```python
from build123d import *

# Parameters (mm, degrees)
SKETCH1_W           = 190
SKETCH1_H           = 29
BOSS_EXTRUDE1_DEPTH = 3
SKETCH2_W           = 190
SKETCH2_H           = 3
BOSS_EXTRUDE2_DEPTH = 3
SKETCH3_W           = 190
SKETCH3_H           = 3
BOSS_EXTRUDE3_DEPTH = 19
SKETCH4_R           = 4.4
BOSS_EXTRUDE4_DEPTH = 190
FILLET1_R           = 1
SKETCH5_W           = 24.6
SKETCH5_H           = 9.5
SKETCH5_W_2         = 22.8
SKETCH5_W_3         = 49.2
CUT_EXTRUDE1_DEPTH  = 99.13898308
CUT_EXTRUDE3_REACH  = 100.139
SKETCH8_R           = 0.79375
CUT_EXTRUDE4_REACH  = 100.139
SKETCH9_W           = 10.2
SKETCH9_H           = 16
DRAFT1_ANGLE        = -5
FILLET2_R           = 5
FILLET3_R           = 2
SKETCH10_R          = 0.79375
BOSS_EXTRUDE5_DEPTH = 3
BOSS_EXTRUDE8_START = -190
SKETCH10_3_R        = 1.75
BOSS_EXTRUDE8_DEPTH = 3
SKETCH12_W          = 26.262284607
SKETCH12_H          = 3
SKETCH12_W_2        = 34.475430786
SKETCH12_W_3        = 52.524569214
CUT_EXTRUDE5_DEPTH  = 105.761807039
SKETCH13_R          = 4.242640687
BOSS_EXTRUDE9_DEPTH = 0.4
FILLET4_R           = 4


with BuildPart() as part:
    # Sketch1 → Boss-Extrude1 (new body)
    with BuildSketch(Plane.XY):
        Rectangle(SKETCH1_W, SKETCH1_H)
    extrude(amount=BOSS_EXTRUDE1_DEPTH)

    # Sketch2 → Boss-Extrude2 (add)
    with BuildSketch(Plane.XY.offset(3)):
        with Locations((0, 13)):
            Rectangle(SKETCH2_W, SKETCH2_H)
    extrude(amount=BOSS_EXTRUDE2_DEPTH)

    # Sketch3 → Boss-Extrude3 (add)
    with BuildSketch(Plane.XY.offset(3)):
        with Locations((0, -13)):
            Rectangle(SKETCH3_W, SKETCH3_H)
    extrude(amount=BOSS_EXTRUDE3_DEPTH)

    # Sketch4 → Boss-Extrude4 (add)
    with BuildSketch(Plane.ZY.offset(95)):
        with Locations((18.5, -9.4)):
            Circle(SKETCH4_R)
    extrude(amount=-BOSS_EXTRUDE4_DEPTH)

    # Fillet1
    fillet1_edges = [part.edges().sort_by_distance(p)[0] for p in [
        (0, -11.5, 14.633477014),
    ]]
    fillet(fillet1_edges, radius=FILLET1_R)

    # Sketch5 → Cut-Extrude1 (cut, through all)
    with BuildSketch(Plane.XY.offset(3)):
        with Locations((-82.7, -9.75)):
            Rectangle(SKETCH5_W, SKETCH5_H)
        with Locations((-47.5, -9.75)):
            Rectangle(SKETCH5_W_2, SKETCH5_H)
        with Locations((0, -9.75)):
            Rectangle(SKETCH5_W_3, SKETCH5_H)
        with Locations((47.5, -9.75)):
            Rectangle(SKETCH5_W_2, SKETCH5_H)
        with Locations((82.7, -9.75)):
            Rectangle(SKETCH5_W, SKETCH5_H)
    extrude(amount=CUT_EXTRUDE1_DEPTH, mode=Mode.SUBTRACT)

    # Sketch8 → Cut-Extrude3 (cut, up to next)
    with BuildSketch(Plane.XY.offset(3), mode=Mode.PRIVATE) as cut_extrude3_sk1:
        with Locations((-12.066777221, -12.066777221)):
            Circle(SKETCH8_R)
    cut_extrude3_tool1 = extrude(cut_extrude3_sk1.sketch, amount=-CUT_EXTRUDE3_REACH, mode=Mode.PRIVATE) & part.part
    # Sketch8 → Cut-Extrude3 (cut, up to next)
    with BuildSketch(Plane.XY.offset(3), mode=Mode.PRIVATE) as cut_extrude3_sk2:
        with Locations((-12.066777221, 12.066777221)):
            Circle(SKETCH8_R)
    cut_extrude3_tool2 = extrude(cut_extrude3_sk2.sketch, amount=-CUT_EXTRUDE3_REACH, mode=Mode.PRIVATE) & part.part
    # Sketch8 → Cut-Extrude3 (cut, up to next)
    with BuildSketch(Plane.XY.offset(3), mode=Mode.PRIVATE) as cut_extrude3_sk3:
        with Locations((12.066777221, 12.066777221)):
            Circle(SKETCH8_R)
    cut_extrude3_tool3 = extrude(cut_extrude3_sk3.sketch, amount=-CUT_EXTRUDE3_REACH, mode=Mode.PRIVATE) & part.part
    # Sketch8 → Cut-Extrude3 (cut, up to next)
    with BuildSketch(Plane.XY.offset(3), mode=Mode.PRIVATE) as cut_extrude3_sk4:
        with Locations((12.066777221, -12.066777221)):
            Circle(SKETCH8_R)
    cut_extrude3_tool4 = extrude(cut_extrude3_sk4.sketch, amount=-CUT_EXTRUDE3_REACH, mode=Mode.PRIVATE) & part.part
    # Sketch8 → Cut-Extrude3 (cut, up to next)
    with BuildSketch(Plane.XY.offset(3), mode=Mode.PRIVATE) as cut_extrude3_sk5:
        Polygon((6.350852961, -11), (12.701705922, 0), (6.350852961, 11), (-6.350852961, 11), (-12.701705922, 0), (-6.350852961, -11), align=None)
    cut_extrude3_tool5 = extrude(cut_extrude3_sk5.sketch, amount=-CUT_EXTRUDE3_REACH, mode=Mode.PRIVATE) & part.part
    add(cut_extrude3_tool1.solids().sort_by_distance((-12.066777, -12.066777, 3))[0], mode=Mode.SUBTRACT)
    add(cut_extrude3_tool2.solids().sort_by_distance((-12.066777, 12.066777, 3))[0], mode=Mode.SUBTRACT)
    add(cut_extrude3_tool3.solids().sort_by_distance((12.066777, 12.066777, 3))[0], mode=Mode.SUBTRACT)
    add(cut_extrude3_tool4.solids().sort_by_distance((12.066777, -12.066777, 3))[0], mode=Mode.SUBTRACT)
    add(cut_extrude3_tool5.solids().sort_by_distance((0, 0, 3))[0], mode=Mode.SUBTRACT)

    # Sketch9 → Cut-Extrude4 (cut, up to next)
    with BuildSketch(Plane.XY.offset(3), mode=Mode.PRIVATE) as cut_extrude4_sk1:
        with Locations((-31.6, 0.9)):
            Rectangle(SKETCH9_W, SKETCH9_H)
    cut_extrude4_tool1 = extrude(cut_extrude4_sk1.sketch, amount=-CUT_EXTRUDE4_REACH, mode=Mode.PRIVATE) & part.part
    # Sketch9 → Cut-Extrude4 (cut, up to next)
    with BuildSketch(Plane.XY.offset(3), mode=Mode.PRIVATE) as cut_extrude4_sk2:
        with Locations((63.4, 0.9)):
            Rectangle(SKETCH9_W, SKETCH9_H)
    cut_extrude4_tool2 = extrude(cut_extrude4_sk2.sketch, amount=-CUT_EXTRUDE4_REACH, mode=Mode.PRIVATE) & part.part
    add(cut_extrude4_tool1.solids().sort_by_distance((-31.6, 0.9, 3))[0], mode=Mode.SUBTRACT)
    add(cut_extrude4_tool2.solids().sort_by_distance((63.4, 0.9, 3))[0], mode=Mode.SUBTRACT)

    # Draft1
    draft1_faces = [part.faces().sort_by_distance(p)[0] for p in [
        (70.4, -10.986471989, 15.250758182),
        (24.6, -10.986471989, 15.250758182),
        (-24.6, -10.986471989, 15.250758182),
        (-70.4, -10.986471989, 15.250758182),
    ]]
    draft(draft1_faces, Plane.XY.offset(22), DRAFT1_ANGLE)

    # Fillet2
    fillet2_edges = [part.edges().sort_by_distance(p)[0] for p in [
        (-58.9, -13, 3),
        (-36.1, -13, 3),
        (58.9, -13, 3),
        (36.1, -13, 3),
    ]]
    fillet(fillet2_edges, radius=FILLET2_R)

    # Fillet3
    fillet3_edges = [part.edges().sort_by_distance(p)[0] for p in [
        (-58.9, -13.283229163, 22),
        (-36.1, -13.283229163, 22),
        (-24.6, -13.283229163, 22),
        (24.6, -13.283229163, 22),
        (58.9, -13.283229163, 22),
        (36.1, -13.283229163, 22),
        (70.4, -13.283229163, 22),
        (-70.4, -13.283229163, 22),
    ]]
    fillet(fillet3_edges, radius=FILLET3_R)

    # Sketch10 → Boss-Extrude5 (add)
    # profile 1 of 2: a face of its own
    with BuildSketch(Plane.ZY.offset(95)):
        Polygon((8.929687245, 14.5), (6, 14.5), (6, 11.5), (3, 11.5), (3, -14.5), (37.070312755, -14.5), (37.070312755, 14.5), align=None)
        with Locations((8.929687245, -12.070312755)):
            Circle(SKETCH10_R, mode=Mode.SUBTRACT)
        with Locations((33.070312755, -12.070312755)):
            Circle(SKETCH10_R, mode=Mode.SUBTRACT)
        with Locations((8.929687245, 12.070312755)):
            Circle(SKETCH10_R, mode=Mode.SUBTRACT)
        Polygon((25.041451884, 7), (29.082903769, 0), (25.041451884, -7), (16.958548116, -7), (12.917096231, 0), (16.958548116, 7), align=None, mode=Mode.SUBTRACT)
        with Locations((33.070312755, 12.070312755)):
            Circle(SKETCH10_R, mode=Mode.SUBTRACT)
    # profile 2 of 2: a face of its own
    with BuildSketch(Plane.ZY.offset(95)):
        Polygon((0, 14.5), (0, -14.5), (3, -14.5), (3, 11.5), (6, 11.5), (6, 14.5), align=None)
    extrude(amount=BOSS_EXTRUDE5_DEPTH)

    # Sketch10<3> → Boss-Extrude8 (add)
    with BuildSketch(Plane.ZY.offset(95).offset(BOSS_EXTRUDE8_START)):
        Polygon((0, 14.5), (8.929687245, 14.5), (37.070312755, 14.5), (37.070312755, -14.5), (0, -14.5), align=None)
        with Locations((21, 0)):
            Circle(SKETCH10_3_R, mode=Mode.SUBTRACT)
    extrude(amount=-BOSS_EXTRUDE8_DEPTH)

    # Sketch12 → Cut-Extrude5 (cut, through all)
    with BuildSketch(Plane.XY.offset(3)):
        with Locations((-81.868857697, 13)):
            Rectangle(SKETCH12_W, SKETCH12_H)
        with Locations((-47.5, 13)):
            Rectangle(SKETCH12_W_2, SKETCH12_H)
        with Locations((0, 13)):
            Rectangle(SKETCH12_W_3, SKETCH12_H)
        with Locations((47.5, 13)):
            Rectangle(SKETCH12_W_2, SKETCH12_H)
        with Locations((81.868857697, 13)):
            Rectangle(SKETCH12_W, SKETCH12_H)
    extrude(amount=CUT_EXTRUDE5_DEPTH, mode=Mode.SUBTRACT)

    # Sketch13 → Boss-Extrude9 (add)
    with BuildSketch(Plane.XZ.offset(14.5)):
        with Locations((-96.5, 37.070312755)):
            Circle(SKETCH13_R)
        with Locations((96.5, 37.070312755)):
            Circle(SKETCH13_R)
        with Locations((98, 0)):
            Circle(SKETCH13_R)
        with Locations((-98, 0)):
            Circle(SKETCH13_R)
    extrude(amount=-BOSS_EXTRUDE9_DEPTH)

    # Fillet4
    fillet4_edges = [part.edges().sort_by_distance(p)[0] for p in [
        (95, 0, 3),
        (-95, 0, 3),
    ]]
    fillet(fillet4_edges, radius=FILLET4_R)


solid = part.part
```
Input: part model. Units: mm. Frame: model coordinates. A direction names the side the tool comes from. Coordinates: 2 decimals unless noted, no trailing zeros. Loops run counter-clockwise (first coordinate to the right, second up) from the corner with the lowest first, then second, coordinate; pieces in that order, holes last. Notation, with made-up numbers: (19, 46) -> (34, 46) arc R26 cw to (34, 61) -> close; hole circle Ø11 at (74, 78). An arc over 180 degrees is marked (long way). Use a Markdown table: item, result.
1) Contact query for flat-ended pins moving along their axis: pin 1 (4 mm diameter, centred on x = 77.5, y = 8, fed in from +Z); pin 2 (10 mm diameter, centred on y = -3.5, z = 28.5, fed in from +X); pin 3 (11 mm diameter, centred on x = 62.5, z = 10, fed in from +Y); pin 4 (1.5 mm diameter, centred on y = 13.5, z = 5, fed in from -X). Output: stop coordinate, or through.
Results found:
| item | result |
|---|---|
| pin 1 | stops at z = 3 |
| pin 2 | stops at x = 98 |
| pin 3 | stops at y = 14.5 |
| pin 4 | stops at x = -98 |
2) Cut plane A-A (x = -49). Return the cut outline in (y, z), then the cut area to 3 significant figures.
Results found:
| item | result |
|---|---|
| outline | (-14.5, 0) -> (14.5, 0) -> (14.5, 3) -> (-14.5, 3) -> close |
| area | 87.0 mm2 |
3) Material intervals for line 1 along X through (y, z) = (-2.25, 8.5); line 2 along Y through (x, z) = (96.95, 21); line 3 along X through (y, z) = (-11.5, 22), sorted ascending. Write a range as from..to.
Results found:
| item | result |
|---|---|
| line 1 | x = -98..-95, 95..98 |
| line 2 | y = -14.5..-1.75, 1.75..14.5 |
| line 3 | x = -98..-95, -70.4..-58.9, -36.1..-24.6, 24.6..36.1, 58.9..70.4, 95..98 |
4) Pull-direction query (X, two-part tool) for faces 5 (the flat face through (-58.9, -11, 17)), 6 (the flat face through (-1, 13, 3)), 7 (the flat face through (98, 0, 19)), 8 (the flat face through (0, 14.5, 2)); classes: released by +X, released by -X, zero draft, split by the parting line, or undercut.
Results found:
| item | result |
|---|---|
| face 5 | undercut |
| face 6 | undercut |
| face 7 | released by +X |
| face 8 | zero draft |
5) Access query for faces 1 (the flat face through (9.48, -5.58, 1.52)), 2 (the flat face through (-96.479, 3.549, 27.034)), 3 (the flat face through (25.21, -10.87, 15.02)), 4 (the flat face through (36.1, -11, 17)). Directions: +Z, -Z, +X, -X, +Y, -Y. A direction counts if a zero-diameter tool reaches every point of the face in a straight line with its end or side. Return the directions, or none.
Results found:
| item | result |
|---|---|
| face 1 | +Z, -Z |
| face 2 | -X |
| face 3 | +Y, -Y |
| face 4 | +Z, +Y, -Y |
